from build123d import *

# Parameters (mm, degrees)
EXTRUDE1_DEPTH                                = 27.94
CBORE_FOR_1_2_SOCKET_HEAD_CAP_SCREW1_AT_COUNT = 2
CBORE_FOR_1_2_SOCKET_HEAD_CAP_SCREW1_AT_PITCH = 109.985226281
CBORE_FOR_1_2_SOCKET_HEAD_CAP_SCREW1_2_COUNT  = 2
CBORE_FOR_1_2_SOCKET_HEAD_CAP_SCREW1_2_PITCH  = 105.596640762
SKETCH6_R                                     = 38.1
CUT_EXTRUDE1_DEPTH                            = 28.94
CUT_EXTRUDE3_DEPTH                            = 81.321852568
CUT_EXTRUDE3_DEPTH_BACK                       = 81.321852568
CUT_EXTRUDE2_DEPTH                            = 1.27
F_1_2_20_TAPPED_HOLE1_D                       = 12.7
F_1_2_20_TAPPED_HOLE1_CSINK_D                 = 15.24
F_1_2_20_TAPPED_HOLE1_CSINK_ANGLE             = 82
SKETCH11_R                                    = 44.45
CUT_EXTRUDE4_DEPTH                            = 1.27
CHAMFER1_SIZE                                 = 0.508


with BuildPart() as part:
    # Sketch1 → Extrude1 (new body)
    with BuildSketch(Plane.XY):
        with BuildLine():
            Line((-25.4, 76.2), (25.4, 76.2))
            ThreePointArc((25.4, 76.2), (80.321852568, 0), (25.4, -76.2))
            Line((25.4, -76.2), (-25.4, -76.2))
            ThreePointArc((-25.4, -76.2), (-80.321852568, 0), (-25.4, 76.2))
        make_face()
    extrude(amount=EXTRUDE1_DEPTH)

    # Sketch3 → CBORE for 1_2 Socket Head Cap Screw1 (revolve, cut)
    with BuildSketch(Plane(origin=(-54.99261314, 31.75, 27.94), x_dir=(0, -1, 0), z_dir=(1, 0, 0))):
        Polygon((0, 0), (0, 27.94), (7.62, 27.94), (6.94563, 27.164226057), (6.94563, 15.24), (10.31875, 15.24), (10.31875, 0.547862954), (10.795, 0), align=None)
    cbore_for_1_2_socket_head_cap_screw1 = revolve(axis=Axis((-54.99261314, 31.75, 34.29), (0, 0, -1)), mode=Mode.SUBTRACT)

    # CBORE for 1_2 Socket Head Cap Screw1 at: CBORE for 1_2 Socket Head Cap Screw1 ×2
    with Locations(*[(i * CBORE_FOR_1_2_SOCKET_HEAD_CAP_SCREW1_AT_PITCH, 0, 0) for i in range(1, CBORE_FOR_1_2_SOCKET_HEAD_CAP_SCREW1_AT_COUNT)]):
        add(cbore_for_1_2_socket_head_cap_screw1, mode=Mode.SUBTRACT)

    # CBORE for 1_2 Socket Head Cap Screw1 2: CBORE for 1_2 Socket Head Cap Screw1 ×2
    with Locations(*[Vector(0.44228869, -0.896872742, 0) * (i * CBORE_FOR_1_2_SOCKET_HEAD_CAP_SCREW1_2_PITCH) for i in range(1, CBORE_FOR_1_2_SOCKET_HEAD_CAP_SCREW1_2_COUNT)]):
        add(cbore_for_1_2_socket_head_cap_screw1, mode=Mode.SUBTRACT)

    # Sketch6 → Cut-Extrude1 (cut, through all)
    with BuildSketch(Plane(origin=(0, 0, 0), x_dir=(-1, 0, 0), z_dir=(0, 0, -1))):
        Circle(SKETCH6_R)
    extrude(amount=-CUT_EXTRUDE1_DEPTH, mode=Mode.SUBTRACT)

    # Sketch10 → Cut-Extrude3 (cut, two sides)
    with BuildSketch(Plane(origin=(0, 0, 0), x_dir=(0, 0, -1), z_dir=(1, 0, 0))) as cut_extrude3_sk:
        with BuildLine():
            Line((0, 6.35), (-9.525, 6.35))
            ThreePointArc((-9.525, 6.35), (-15.875, 0), (-9.525, -6.35))
            Line((-9.525, -6.35), (0, -6.35))
            Line((0, -6.35), (0, 6.35))
        make_face()
    extrude(amount=CUT_EXTRUDE3_DEPTH, mode=Mode.SUBTRACT)
    extrude(cut_extrude3_sk.sketch, amount=-CUT_EXTRUDE3_DEPTH_BACK, mode=Mode.SUBTRACT)

    # Sketch9 → Cut-Extrude2 (cut)
    with BuildSketch(Plane(origin=(0, 0, 0), x_dir=(-1, 0, 0), z_dir=(0, 0, -1))):
        with BuildLine():
            Line((-79.634687985, 10.484105568), (-37.774049218, 4.973047924))
            ThreePointArc((-37.774049218, 4.973047924), (-32.995567884, -19.05), (-14.580238773, -35.199810189))
            Line((-14.580238773, -35.199810189), (-30.737842235, -74.207715601))
            ThreePointArc((-30.737842235, -74.207715601), (-69.560764803, -40.160926284), (-79.634687985, 10.484105568))
        make_face()
        with BuildLine():
            Line((-48.89684575, 63.723610033), (-23.193810445, 30.226762265))
            ThreePointArc((-23.193810445, 30.226762265), (0, 38.1), (23.193810445, 30.226762265))
            Line((23.193810445, 30.226762265), (48.89684575, 63.723610033))
            ThreePointArc((48.89684575, 63.723610033), (0, 80.321852568), (-48.89684575, 63.723610033))
        make_face()
        with BuildLine():
            Line((37.774049218, 4.973047924), (79.634687985, 10.484105568))
            ThreePointArc((79.634687985, 10.484105568), (69.560764803, -40.160926284), (30.737842235, -74.207715601))
            Line((30.737842235, -74.207715601), (14.580238773, -35.199810189))
            ThreePointArc((14.580238773, -35.199810189), (32.995567884, -19.05), (37.774049218, 4.973047924))
        make_face()
    extrude(amount=-CUT_EXTRUDE2_DEPTH, mode=Mode.SUBTRACT)

    # 1_2-20 Tapped Hole1 (through all)
    with Locations(Plane.XY.offset(27.94)):
        with Locations((0, 50.8), (-43.994090512, -25.4), (43.994090512, -25.4)):
            CounterSinkHole(F_1_2_20_TAPPED_HOLE1_D / 2, F_1_2_20_TAPPED_HOLE1_CSINK_D / 2, counter_sink_angle=F_1_2_20_TAPPED_HOLE1_CSINK_ANGLE)

    # Sketch11 → Cut-Extrude4 (cut)
    with BuildSketch(Plane(origin=(0, 0, 0), x_dir=(-1, 0, 0), z_dir=(0, 0, -1))):
        Circle(SKETCH11_R)
    extrude(amount=-CUT_EXTRUDE4_DEPTH, mode=Mode.SUBTRACT)

    # Chamfer1
    chamfer1_edges = [part.edges().sort_by_distance(p)[0] for p in [
        (-28.086591676, -75.251201771, 0),
        (-69.560764803, 40.160926284, 0),
        (0, -76.2, 0),
        (-37.978145635, 49.494083005, 0),
        (-38.355757488, 22.464157396, 0),
        (-46.113564564, 6.35, 0),
        (-63.9338633, 8.417052784, 0),
        (46.113564564, 6.35, 0),
        (38.355757488, 22.464157396, 0),
        (37.978145635, 49.494083005, 0),
        (63.9338633, 8.417052784, 0),
        (69.560764803, 40.160926284, 0),
        (0, -44.45, 0),
        (23.874060402, -57.637080411, 0),
        (-23.874060402, -57.637080411, 0),
        (28.086591676, -75.251201771, 0),
    ]]
    chamfer(chamfer1_edges, length=CHAMFER1_SIZE)


solid = part.part
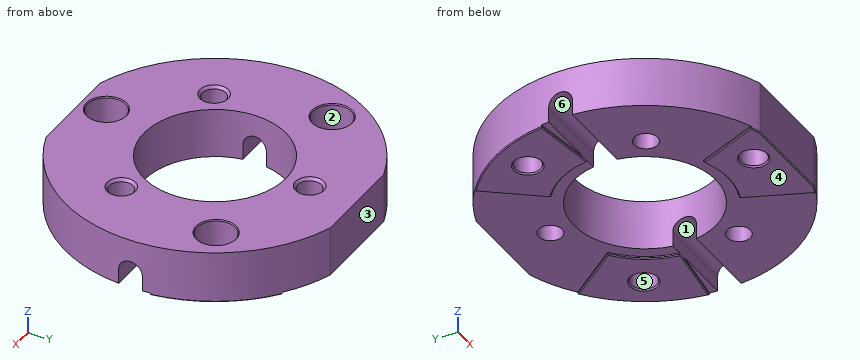
Work out the finished part from the listing and answer in its coordinate system (mm). Face numbers are marked on the shaded views. A direction names the side the tool comes from. Give positions to 0.01 mm unless a question says otherwise; leave off trailing zeros. Order: outer loops, then holes, each group sorted by start corner. A loop starts at its lowest first (then second) coordinate and runs counter-clockwise, first axis right, second up. Notation, with made-up numbers: M 37,-11 L 67,-11 A16 cw 67,10 Z; hole C 12,-2.5 d11. An arc over 180 degrees is marked long. Return JSON: item names as keys, results as strings.
Q1. Find the intervals of material crossed by line 1 along Y through (x, z) = (0, 17.75); line 2 along Y through (x, z) = (5, 3.5); line 3 along Y through (x, z) = (-4.5, 6.75), in increasing order. Write a range as [from, to].
Answer below:
{"line 1": "y = [-76.2, -69.1], [-56.81, -38.1], [38.1, 44.45], [57.15, 76.2]", "line 2": "y = [-76.2, -37.77], [37.77, 46.89], [54.71, 76.2]", "line 3": "y = [-76.2, -68.78], [-57.14, -37.83], [37.83, 46.32], [55.28, 76.2]"}
Q2. Each of these flat-tipped pins is pushed along its axis until it touches: pin 1 (4 mm diameter, centred on y = 13, z = 14, fed in from +X); pin 2 (16.5 mm diameter, centred on x = -43.99, y = -25.4, fed in from +Z); pin 3 (4 mm diameter, centred on x = -53, z = 24.5, fed in from -Y); pin 4 (5 mm diameter, centred on y = -5, z = 8, fed in from -X). Where does it stop, or does it pass through?
Answer below:
{"pin 1": "stops at x = 79.57", "pin 2": "stops at z = 27.94", "pin 3": "stops at y = -62.05", "pin 4": "stops at x = -80.07"}
Q3. The mould has two halves that part along Y. Classify the marked faces 3, 4, 5 and 6: pulls with the +Y half, pulls with the -Y half, needs draft (parallel to the pull), parting line crosses it, or undercut.
Answer below:
{"face 3": "pulls with the +Y half", "face 4": "needs draft", "face 5": "undercut", "face 6": "undercut"}
Q4. Which of the six approach directions +Z, -Z, +X, -X, +Y, -Y give full straight-line access (tool end or side, diameter ignored) to the marked faces 1 and 2?
Answer below:
{"face 1": "-Z, +X, -X", "face 2": "+Z"}
Q5. Find section A-A, the plane y = -25.4. Write down the section's boundary in (x, z), and give its area (3 significant figures).
Answer below:
{"outline": "M -76.2,1.27 L -50.34,1.27 L -50.34,26.48 L -51.61,27.94 L -76.2,27.94 Z; M -37.64,1.27 L -28.4,1.27 L -28.4,27.94 L -36.37,27.94 L -37.64,26.48 Z; M 28.4,1.27 L 37.64,1.27 L 37.64,26.48 L 36.37,27.94 L 28.4,27.94 Z; M 50.34,1.27 L 76.2,1.27 L 76.2,27.94 L 51.61,27.94 L 50.34,26.48 Z", "area": "1,870 mm^2"}
Q6. Find section B-B, the plane z = 21.75. Write down the section's boundary in (x, y).
Answer below:
{"outline": "M -25.4,-76.2 L 25.4,-76.2 A80.32 ccw 25.4,76.2 L -25.4,76.2 A80.32 ccw Z; hole C -54.99,31.75 d20.64; hole C -43.99,-25.4 d12.7; hole C 0,0 d76.2; hole C -8.29,-62.96 d20.64; hole C 0,50.8 d12.7; hole C 43.99,-25.4 d12.7; hole C 54.99,31.75 d20.64"}
